The listing builds one solid part. Answer for the finished solid, in the listing's coordinates (mm). Give positions to 0.01 mm unless a question says otherwise; leave off trailing zeros. Loops run counter-clockwise (first coordinate to the right, second up) from the corner with the lowest first, then second, coordinate; pieces in that order, holes last. Notation, with made-up numbers: M 89,-1.75 L 132,-1.75 A26 cw 132,21.25 Z; hole C 28.5,-8 d5. An arc over 180 degrees is marked long. One line per item, written item: value. Start each with the question number.
Q1. Flat-ended cylindrical pins translate along their axes: pin 1 (3.5 mm diameter, centred on x = 40, y = 2, fed in from +Z); pin 2 (1.5 mm diameter, centred on y = 67, z = 3, fed in from +X); pin 3 (2 mm diameter, centred on x = -32, z = 1.5, fed in from -Y). Find the tip coordinate at first contact, or state that the pin passes through.
Q2. A cutting plane is placed at D-D, the plane y = -65. Determine the outline of the cut face in (x, z).
Q3. Consider L1, parallel to Y at x = 40, z = 2.15 (3 decimals); L2, parallel to Y at x = 0, z = 1.5 (3 decimals); L3, parallel to Y at x = -8.5, z = 1.5 (3 decimals). Determine where each line is inside the solid, lowest interval first.
Q4. A cutting plane is placed at B-B, the plane z = 0.8. State how many separate pieces and enclosed holes the cut face has, and give its area (3 significant figures).
Q5. A cutting plane is placed at A-A, the plane y = -6. Determine the outline of the cut face in (x, z), and give its area (4 significant figures).
Q6. A cutting plane is placed at C-C, the plane y = -39. Determine the outline of the cut face in (x, z).
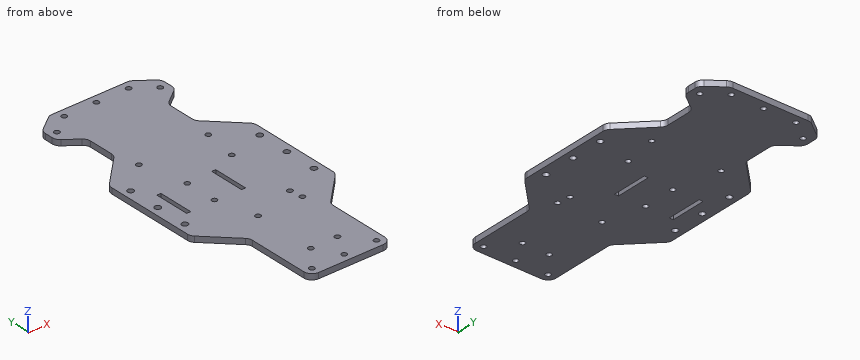
from build123d import *

# Parameters (mm, degrees)
F0_R     = 1.625
F0_R_2   = 1.875
F0_W     = 2.5
F0_H     = 22
F1_DEPTH = 3.5
F2_R     = 5


# Not quite as in the source:
# - a feature names something its author has since deleted; it is built from what else it names


with BuildPart() as f1:
    # F0 (on Top) → F1 (new body)
    with BuildSketch(Plane.XY):
        with BuildLine():
            Line((-25, 52), (-45, 32))
            Line((-45, 32), (-45, -28))
            Line((-45, -28), (-25, -48))
            Line((-25, -48), (-25, -88))
            ThreePointArc((-25, -88), (-23.5355339059, -91.5355339059), (-20, -93))
            Line((-20, -93), (20, -93))
            ThreePointArc((20, -93), (23.5355339059, -91.5355339059), (25, -88))
            Line((25, -88), (25, -48))
            Line((25, -48), (45, -28))
            Line((45, -28), (45, 32))
            Line((45, 32), (25, 52))
            Line((25, 52), (25, 72))
            Line((25, 72), (37, 81))
            Line((37, 81), (37, 91))
            Line((37, 91), (25, 100))
            Line((25, 100), (-25, 100))
            Line((-25, 100), (-37, 91))
            Line((-37, 91), (-37, 81))
            Line((-37, 81), (-25, 72))
            Line((-25, 72), (-25, 52))
        make_face()
        with Locations((-20, -88)):
            Circle(F0_R, mode=Mode.SUBTRACT)
        with Locations((-8.5, -73.5)):
            Circle(F0_R, mode=Mode.SUBTRACT)
        with Locations((-40, -18)):
            Circle(F0_R_2, mode=Mode.SUBTRACT)
        with Locations((-40, 2)):
            Circle(F0_R_2, mode=Mode.SUBTRACT)
        with Locations((-31.75, 0)):
            Rectangle(F0_W, F0_H, mode=Mode.SUBTRACT)
        with Locations((-8.5, -34.5)):
            Circle(F0_R, mode=Mode.SUBTRACT)
        with Locations((-15, -10)):
            Circle(F0_R, mode=Mode.SUBTRACT)
        with Locations((0, -88)):
            Circle(F0_R, mode=Mode.SUBTRACT)
        with Locations((8, -73.5)):
            Circle(F0_R, mode=Mode.SUBTRACT)
        with Locations((20, -88)):
            Circle(F0_R, mode=Mode.SUBTRACT)
        with Locations((19, -34.5)):
            Circle(F0_R, mode=Mode.SUBTRACT)
        with Locations((18, -26.5)):
            Circle(F0_R, mode=Mode.SUBTRACT)
        with Locations((2.25, 0)):
            Rectangle(F0_W, F0_H, mode=Mode.SUBTRACT)
        with Locations((40, -18)):
            Circle(F0_R_2, mode=Mode.SUBTRACT)
        with Locations((40, 2)):
            Circle(F0_R_2, mode=Mode.SUBTRACT)
        with Locations((-40, 22)):
            Circle(F0_R_2, mode=Mode.SUBTRACT)
        with Locations((-15, 10)):
            Circle(F0_R, mode=Mode.SUBTRACT)
        with Locations((-21.5, 38)):
            Circle(F0_R, mode=Mode.SUBTRACT)
        with Locations((-32, 86)):
            Circle(F0_R, mode=Mode.SUBTRACT)
        with Locations((-20, 95)):
            Circle(F0_R, mode=Mode.SUBTRACT)
        with Locations((18, 16.5)):
            Circle(F0_R, mode=Mode.SUBTRACT)
        with Locations((21.5, 38)):
            Circle(F0_R, mode=Mode.SUBTRACT)
        with Locations((40, 22)):
            Circle(F0_R_2, mode=Mode.SUBTRACT)
        with Locations((0, 95)):
            Circle(F0_R, mode=Mode.SUBTRACT)
        with Locations((20, 95)):
            Circle(F0_R, mode=Mode.SUBTRACT)
        with Locations((32, 86)):
            Circle(F0_R, mode=Mode.SUBTRACT)
    extrude(amount=F1_DEPTH)

    # F2
    f2_edges = [f1.edges().sort_by_distance(p)[0] for p in [
        (-45, -28, 1.75),
        (-25, -48, 1.75),
        (25, -48, 1.75),
        (45, -28, 1.75),
        (45, 32, 1.75),
        (25, 52, 1.75),
        (25, 72, 1.75),
        (-25, 52, 1.75),
        (-45, 32, 1.75),
        (-25, 72, 1.75),
        (-37, 81, 1.75),
        (-37, 91, 1.75),
        (-25, 100, 1.75),
        (25, 100, 1.75),
        (37, 91, 1.75),
        (37, 81, 1.75),
    ]]
    fillet(f2_edges, radius=F2_R)


solid = f1.part
Answer block:
1. pin 1: through
1. pin 2: x = 25
1. pin 3: y = -42
2. outline: M -25,0 L 25,0 L 25,3.5 L -25,3.5 Z
3. L1: -33 to -19.875, -16.125 to 0.125, 3.875 to 20.125, 23.875 to 37
3. L2: -93 to -89.625, -86.375 to 93.375, 96.625 to 100
3. L3: -93 to -75.125, -71.875 to -36.125, -32.875 to 100
4. separate pieces: 1
4. enclosed holes: 26
4. area: 13,000 mm^2
5. outline: M -45,0 L -33,0 L -33,3.5 L -45,3.5 Z; M -30.5,0 L 1,0 L 1,3.5 L -30.5,3.5 Z; M 3.5,0 L 45,0 L 45,3.5 L 3.5,3.5 Z
5. area: 297.5 mm^2
6. outline: M -34,0 L 34,0 L 34,3.5 L -34,3.5 Z
